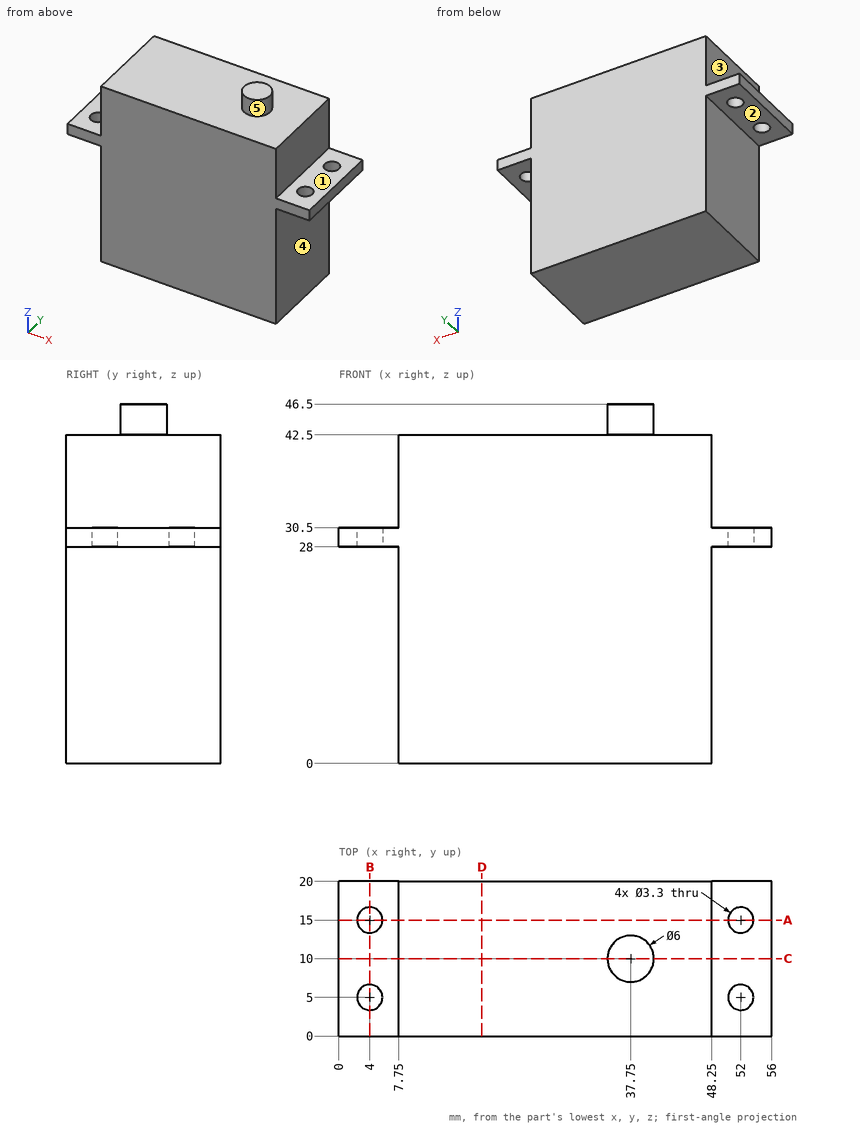
Part print with two shaded views. Sizes in mm from the minimum x, y, z corner. A direction names the side the tool comes from. Coordinates: 2 decimals unless noted, no trailing zeros. Write each loop counter-clockwise with the first axis right and the second up, starting at its lowest first coordinate (ties: lowest second). Pieces come first, ordered by that corner, then holes.
(1) 3-axis set-ups, long thin cutter, end or side, ignore diameter. For the marked faces 1, 2, 3, 4 and 5: which of +Z, -Z, +X, -X, +Y, -Y reach the whole face in a straight line?
(2) Cut at A-A on y = 15. List the corners of the cut face in (x, z), and give its area (3 significant figures).
(3) Cut at B-B on x = 4. List the corners of the cut face in (y, z), and give its area (3 significant figures).
(4) Cut at C-C on y = 10. List the corners of the cut face in (x, z), and give its area (3 significant figures).
(5) Pin check, flat tips, straight feed: pin 1 Ø8.5 at (x, y) = (50.5, 7.5) entering from -Z; pin 2 Ø6 at (y, z) = (8, 24) entering from +X; pin 3 Ø2.5 at (x, y) = (3, 5) entering from -Z; pin 4 Ø10 at (x, y) = (16.5, 15) entering from +Z. Stop position of each tip, or through.
(6) Cut at D-D on x = 18.5. List the corners of the cut face in (y, z), and give its area (3 significant figures).
(7) Drill centre lines: line 1 (Y direction, x = 52, z = 29.8); line 2 (X direction, y = 6.5, z = 8); line 3 (Z direction, x = 25.5, y = 6.75). Where is each one in solid material? Low to high.
Working result:
1. face 1: +Z, +X, +Y, -Y
1. face 2: -Z, -X, +Y, -Y
1. face 3: +Z, -X, +Y, -Y
1. face 4: -Z, +X, +Y, -Y
1. face 5: +Z
2. outline: (0, 28) - (2.35, 28) - (2.35, 30.5) - (0, 30.5) - close; (5.65, 28) - (7.75, 28) - (7.75, 0) - (48.25, 0) - (48.25, 28) - (50.35, 28) - (50.35, 30.5) - (48.25, 30.5) - (48.25, 42.5) - (7.75, 42.5) - (7.75, 30.5) - (5.65, 30.5) - close; (53.65, 28) - (56, 28) - (56, 30.5) - (53.65, 30.5) - close
2. area: 1,740 mm2
3. outline: (0, 28) - (3.35, 28) - (3.35, 30.5) - (0, 30.5) - close; (6.65, 28) - (13.35, 28) - (13.35, 30.5) - (6.65, 30.5) - close; (16.65, 28) - (20, 28) - (20, 30.5) - (16.65, 30.5) - close
3. area: 33.5 mm2
4. outline: (0, 28) - (7.75, 28) - (7.75, 0) - (48.25, 0) - (48.25, 28) - (56, 28) - (56, 30.5) - (48.25, 30.5) - (48.25, 42.5) - (40.75, 42.5) - (40.75, 46.5) - (34.75, 46.5) - (34.75, 42.5) - (7.75, 42.5) - (7.75, 30.5) - (0, 30.5) - close
4. area: 1,780 mm2
5. pin 1: stops at z = 0
5. pin 2: stops at x = 48.25
5. pin 3: stops at z = 28
5. pin 4: stops at z = 42.5
6. outline: (0, 0) - (20, 0) - (20, 42.5) - (0, 42.5) - close
6. area: 850 mm2
7. line 1: y = 0 to 3.35, 6.65 to 13.35, 16.65 to 20
7. line 2: x = 7.75 to 48.25
7. line 3: z = 0 to 42.5
